Can you work these out from the model? Positions are in its coordinate system, mm. Face numbers are marked on the shaded views. A direction names the side the tool comes from. Give positions to 0.01 mm unless a question says otherwise; leave off trailing zeros. Write each loop counter-clockwise with the first axis right and the second up, starting at its lowest first coordinate (ties: lowest second). Pieces come first, ordered by that corner, then holes. Notation, with made-up numbers: M 13,32 L 59,32 A26 cw 59,68 Z; hole C 73,-1.75 d4. An arc over 180 degrees is marked long. Write each question's results on one line, items separated by ' | '.
from build123d import *

# Parameters (mm, degrees)
M4X0_7_TAPPED_HOLE1_D = 3.3
CIRPATTERN1_COUNT     = 6


with BuildPart() as part:
    # Sketch1 → Revolve1 (revolve)
    with BuildSketch(Plane(origin=(0, 0, 0), x_dir=(0, 0, -1), z_dir=(1, 0, 0)), mode=Mode.PRIVATE) as revolve1_sk:
        Polygon((0, 31.75), (-9.155682966, 31.75), (-10, 30.2876), (-10, 28.575), (-15, 28.575), (-15, 21), (0, 21), align=None)
    revolve(revolve1_sk.sketch.rotate(Axis((0, 0, 15), (0, 0, -1)), 90), axis=Axis((0, 0, 15), (0, 0, -1)))

    # M4x0.7 Tapped Hole1 (through all)
    with Locations(Plane(origin=(0, 0, 0), x_dir=(-1, 0, 0), z_dir=(0, 0, -1))):
        with Locations((0, 24.75)):
            m4x0_7_tapped_hole1 = Hole(M4X0_7_TAPPED_HOLE1_D / 2)

    # CirPattern1: M4x0.7 Tapped Hole1 ×6 about axis
    cirpattern1_axis = Axis((0, 0, 0), (0, 0, 1))
    for i in range(1, CIRPATTERN1_COUNT):
        add(m4x0_7_tapped_hole1.rotate(cirpattern1_axis, i * 360 / CIRPATTERN1_COUNT), mode=Mode.SUBTRACT)


solid = part.part
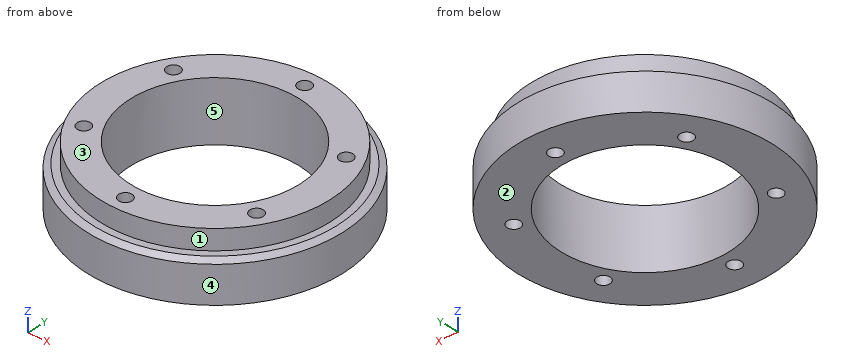
Item 1: Thinking about a two-plate mould opening in X: for the marked faces 3, 4 and 5, which applies, +X half, -X half, draft (parallel to the pull), parting line (faces both ways), or undercut?
Geometry says:
face 3: draft | face 4: parting line | face 5: undercut
Item 2: I'm going to push flat-ended pins straight in: pin 1 (4.5 mm diameter, centred on x = 0, y = -24.75, fed in from -Z); pin 2 (3 mm diameter, centred on x = -17, z = 5.5, fed in from +Y); pin 3 (1 mm diameter, centred on y = -2, z = 4.5, fed in from +X); pin 4 (6 mm diameter, centred on x = -10.5, z = 8, fed in from -Y). Where does each tip first touch, or does it pass through?
Geometry says:
pin 1: stops at z = 0 | pin 2: stops at y = 27.71 | pin 3: stops at x = 31.71 | pin 4: stops at y = -30.85
Item 3: I want a section at B-B, the plane z = 11.5. Please give me the cut outline in (x, y) (3 decimals), and give its area (3 significant figures).
Geometry says:
outline: C 0,0 d57.15; hole C -21.434,-12.375 d3.3; hole C -21.434,12.375 d3.3; hole C 0,0 d42; hole C 0,-24.75 d3.3; hole C 0,24.75 d3.3; hole C 21.434,-12.375 d3.3; hole C 21.434,12.375 d3.3 | area: 1,130 mm2
Item 4: I want a section at C-C, the plane z = 5. Please give me the cut outline in (x, y) (3 decimals), and give its area (3 significant figures).
Geometry says:
outline: C 0,0 d63.5; hole C -21.434,-12.375 d3.3; hole C -21.434,12.375 d3.3; hole C 0,0 d42; hole C 0,-24.75 d3.3; hole C 0,24.75 d3.3; hole C 21.434,-12.375 d3.3; hole C 21.434,12.375 d3.3 | area: 1,730 mm2
Item 5: If I drill on line 1 (Y direction, x = 0, z = 5.5); line 2 (Y direction, x = 9.5, z = 9); line 3 (Y direction, x = 9.5, z = 14.25), over which ranges is the centre line in solid material (lowest first)? Write a range as from..to.
Geometry says:
line 1: y = -31.75..-26.4, -23.1..-21, 21..23.1, 26.4..31.75 | line 2: y = -30.3..-18.73, 18.73..30.3 | line 3: y = -26.95..-18.73, 18.73..26.95
Item 6: I want a section at A-A, the plane x = 0. Please give me the cut outline in (y, z) (3 decimals), and give its area (3 significant figures).
Geometry says:
outline: M -31.75,0 L -26.4,0 L -26.4,15 L -28.575,15 L -28.575,10 L -30.288,10 L -31.75,9.156 Z; M -23.1,0 L -21,0 L -21,15 L -23.1,15 Z; M 21,0 L 23.1,0 L 23.1,15 L 21,15 Z; M 26.4,0 L 31.75,0 L 31.75,9.156 L 30.288,10 L 28.575,10 L 28.575,15 L 26.4,15 Z | area: 191 mm2
Item 7: For the marked faces 1 and 2, which set-ups out of +Z, -Z, +X, -X, +Y, -Y let a thin tool reach every point of the face, with its end or its side?
Geometry says:
face 1: +Z | face 2: -Z, +X, -X, +Y, -Y
